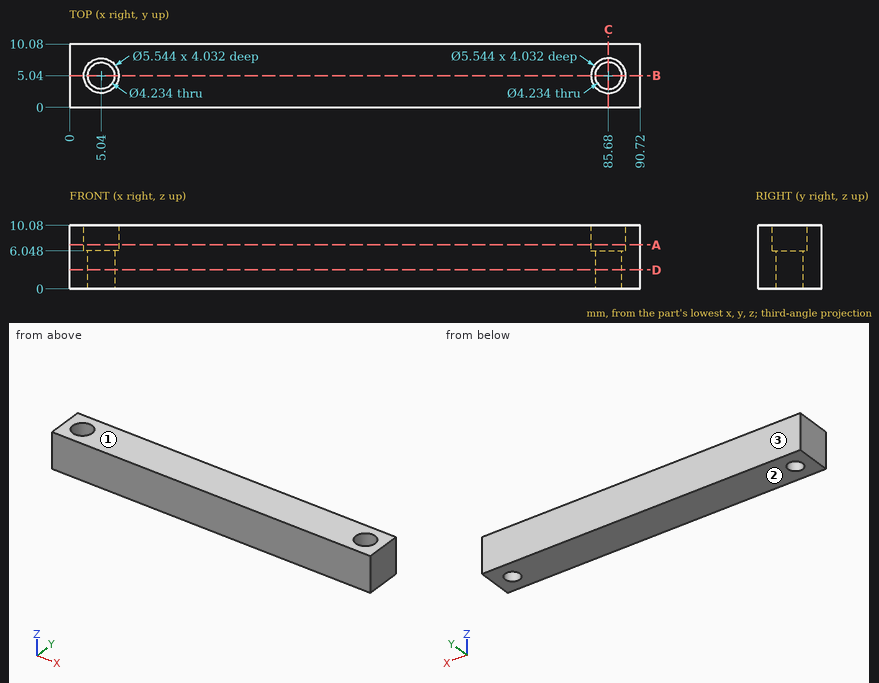
Job drawing, mm, ordinate dimensions from the low corner. One solid piece. Coordinates: 2 decimals unless noted, no trailing zeros. Write each loop counter-clockwise with the first axis right and the second up, starting at its lowest first coordinate (ties: lowest second). Pieces come first, ordered by that corner, then holes.
Item 1: Slice it at A-A (z = 7). Write the cut outline in (x, y).
Item 2: Pin check, flat tips, straight feed: pin 1 (4.5 mm diameter, centred on x = 85.68, y = 5.04, fed in from +Z); pin 2 (4 mm diameter, centred on x = 5.04, y = 5.04, fed in from -Z). Stop position of each tip, or through.
Item 3: Slice it at D-D (z = 3). Write the cut outline in (x, y).
Item 4: Probe line 1 (X direction, y = 5.04, z = 8.6); line 2 (X direction, y = 5.04, z = 2.25); line 3 (Y direction, x = 5.04, z = 7.3). List the from-to ranges inside material, lowest first.
Item 5: Slice it at B-B (y = 5.04). Write the cut outline in (x, z).
Item 6: Slice it at C-C (x = 85.68). Write the cut outline in (y, z).
Item 7: Mould opens along Z. For the marked faces 1, 2 and 3 say: released by +Z, released by -Z, zero draft, split by the parting line, or undercut.
Results found:
1. outline: (0, 0) - (90.72, 0) - (90.72, 10.08) - (0, 10.08) - close; hole circle Ø5.54 at (5.04, 5.04); hole circle Ø5.54 at (85.68, 5.04)
2. pin 1: stops at z = 6.05
2. pin 2: passes through
3. outline: (0, 0) - (90.72, 0) - (90.72, 10.08) - (0, 10.08) - close; hole circle Ø4.23 at (5.04, 5.04); hole circle Ø4.23 at (85.68, 5.04)
4. line 1: x = 0 to 2.27, 7.81 to 82.91, 88.45 to 90.72
4. line 2: x = 0 to 2.92, 7.16 to 83.56, 87.8 to 90.72
4. line 3: y = 0 to 2.27, 7.81 to 10.08
5. outline: (0, 0) - (2.92, 0) - (2.92, 6.05) - (2.27, 6.05) - (2.27, 10.08) - (0, 10.08) - close; (7.16, 0) - (83.56, 0) - (83.56, 6.05) - (82.91, 6.05) - (82.91, 10.08) - (7.81, 10.08) - (7.81, 6.05) - (7.16, 6.05) - close; (87.8, 0) - (90.72, 0) - (90.72, 10.08) - (88.45, 10.08) - (88.45, 6.05) - (87.8, 6.05) - close
6. outline: (0, 0) - (2.92, 0) - (2.92, 6.05) - (2.27, 6.05) - (2.27, 10.08) - (0, 10.08) - close; (7.16, 0) - (10.08, 0) - (10.08, 10.08) - (7.81, 10.08) - (7.81, 6.05) - (7.16, 6.05) - close
7. face 1: released by +Z
7. face 2: released by -Z
7. face 3: zero draft
